Read the model definition and answer for the solid it produces. Units are mm, in the model's axes. A direction names the side the tool comes from. Coordinates: 2 decimals unless noted, no trailing zeros. Loops run counter-clockwise (first coordinate to the right, second up) from the corner with the lowest first, then second, coordinate; pieces in that order, holes last.
from build123d import *

# Parameters (mm, degrees)
SKETCH1_W           = 31
SKETCH1_H           = 45.4
BOSS_EXTRUDE1_DEPTH = 12
SKETCH2_W           = 27
SKETCH2_H           = 10
CUT_EXTRUDE1_DEPTH  = 57.268641356
SKETCH3_R           = 1.6
CUT_EXTRUDE2_DEPTH  = 10
SKETCH4_W           = 15
SKETCH4_H           = 12
BOSS_EXTRUDE2_DEPTH = 15
SKETCH5_R           = 1.6
CUT_EXTRUDE3_DEPTH  = 20
FILLET1_R           = 5
BOSS_EXTRUDE3_DEPTH = 15
CHAMFER1_SIZE       = 5
CUT_EXTRUDE4_DEPTH  = 4


with BuildPart() as part:
    # Sketch1 → Boss-Extrude1 (new body)
    with BuildSketch(Plane(origin=(0, 0, 0), x_dir=(1, 0, 0), z_dir=(0, 1, 0))):
        with Locations((15.5, 22.7)):
            Rectangle(SKETCH1_W, SKETCH1_H)
    extrude(amount=BOSS_EXTRUDE1_DEPTH)

    # Sketch2 → Cut-Extrude1 (cut, through all)
    with BuildSketch(Plane.XY):
        with Locations((15.5, 5)):
            Rectangle(SKETCH2_W, SKETCH2_H)
    extrude(amount=-CUT_EXTRUDE1_DEPTH, mode=Mode.SUBTRACT)

    # Sketch3 → Cut-Extrude2 (cut)
    with BuildSketch(Plane(origin=(0, 12, 0), x_dir=(1, 0, 0), z_dir=(0, 1, 0))):
        with Locations(Location((5.5, 32.7, 0), (0, 0, 270))):
            Circle(SKETCH3_R)
        with Locations(Location((25.5, 32.7, 0), (0, 0, 270))):
            Circle(SKETCH3_R)
        with Locations(Location((25.5, 12.7, 0), (0, 0, 270))):
            Circle(SKETCH3_R)
        with Locations(Location((5.5, 12.7, 0), (0, 0, 270))):
            Circle(SKETCH3_R)
    extrude(amount=-CUT_EXTRUDE2_DEPTH, mode=Mode.SUBTRACT)

    # Sketch4 → Boss-Extrude2 (add)
    with BuildSketch(Plane.ZY):
        with Locations((-7.5, 6)):
            Rectangle(SKETCH4_W, SKETCH4_H)
    extrude(amount=BOSS_EXTRUDE2_DEPTH)

    # Sketch5 → Cut-Extrude3 (cut)
    with BuildSketch(Plane(origin=(0, 12, 0), x_dir=(1, 0, 0), z_dir=(0, 1, 0))):
        with Locations(Location((-10, 5, 0), (0, 0, 270))):
            Circle(SKETCH5_R)
    extrude(amount=-CUT_EXTRUDE3_DEPTH, mode=Mode.SUBTRACT)

    # Fillet1
    fillet1_edges = [part.edges().sort_by_distance(p)[0] for p in [
        (-15, 6, -15),
        (-15, 6, 0),
    ]]
    fillet(fillet1_edges, radius=FILLET1_R)

    # Sketch6 → Boss-Extrude3 (add)
    with BuildSketch(Plane(origin=(31, 0, 0), x_dir=(0, 0, -1), z_dir=(1, 0, 0))):
        Polygon((5, 0), (10, 0), (10, 4.7), (25, 4.7), (25, 0), (30, 0), (30, 12), (5, 12), align=None)
    extrude(amount=BOSS_EXTRUDE3_DEPTH)

    # Chamfer1
    chamfer1_edges = [part.edges().sort_by_distance(p)[0] for p in [
        (38.5, 0, -5),
        (38.5, 0, -30),
    ]]
    chamfer(chamfer1_edges, length=CHAMFER1_SIZE - 0.0001)  # a hair under: the kernel refuses the full size

    # Sketch7 → Cut-Extrude4 (cut)
    with BuildSketch(Plane(origin=(43, 0, 0), x_dir=(0, 0, -1), z_dir=(1, 0, 0))):
        Polygon((5, 7), (15, 12), (5, 12), align=None)
        Polygon((30, 7), (20, 12), (30, 12), align=None)
    extrude(amount=-CUT_EXTRUDE4_DEPTH, mode=Mode.SUBTRACT)


with BuildPart() as body_2:
    # Mirror2: mirrored copy
    add(part.part.mirror(Plane(origin=(31, 12, 0), x_dir=(0, 0, 1), z_dir=(-1, 0, 0))))


with BuildPart() as body_3:
    # Mirror3: mirrored copy
    add(body_2.part.mirror(Plane(origin=(62, 12, -45.4), x_dir=(1, 0, 0), z_dir=(0, 0, 1))))


solid = body_3.part
Item 1: Find the intervals of material crossed by line 1 along Z through (x, y) = (36.5, 11.5); line 2 along X through (y, z) = (9.5, -64); line 3 along X through (y, z) = (2.75, -68.5), in increasing order.
Numbers:
line 1: z = -90.8 to -79.7, -76.5 to -59.7, -56.5 to -45.4
line 2: x = 16 to 19, 23 to 33, 60 to 62
line 3: x = 31 to 33, 60 to 62
Item 2: A cutting plane is placed at A-A on x = 56.5. Determine the outline of the cut face in (y, z), then the cut area to 3 significant figures.
Numbers:
outline: (10, -90.8) - (12, -90.8) - (12, -79.7) - (10, -79.7) - close; (10, -76.5) - (12, -76.5) - (12, -59.7) - (10, -59.7) - close; (10, -56.5) - (12, -56.5) - (12, -45.4) - (10, -45.4) - close
area: 78.0 mm2
Item 3: Which of the six approach directions +Z, -Z, +X, -X, +Y, -Y give full straight-line access (tool end or side, diameter ignored) to faces 1 (the face through (24, 8, -60.8)), 2 (the face through (20.972, 9.465, -65.73)), 3 (the face through (23.6, 2.5, -63.3)), 4 (the face through (23.6, 2.5, -83.3))?
Numbers:
face 1: +Z, -X, +Y, -Y
face 2: +Z, +Y
face 3: +Z, -X, -Y
face 4: -Z, -X, -Y
Item 4: A cutting plane is placed at B-B on z = -74.5. Determine the outline of the cut face in (x, y), then the cut area to 4 significant figures.
Numbers:
outline: (16, 4.7) - (31, 4.7) - (31, 0) - (33, 0) - (33, 10) - (60, 10) - (60, 0) - (62, 0) - (62, 12) - (16, 12) - close
area: 211.5 mm2
Item 5: Determine the mould class of faces 5 (the face through (75.57, 6.08, -89.3)), 6 (the face through (60, 5, -68)), 7 (the face through (45.4, 10.4, -45.4)), 8 (the face through (56.019, 11.014, -79.626)) for opening direction X: released by +X, released by -X, zero draft, split by the parting line, or undercut.
Numbers:
face 5: released by +X
face 6: undercut
face 7: zero draft
face 8: undercut
Item 6: Given pin 1 (2.5 mm diameter, centred on x = 24, y = 3, fed in from -Z); pin 2 (1.9 mm diameter, centred on x = 36.5, z = -78.1, fed in from -Y); pin 3 (5 mm diameter, centred on x = 69, y = 7.5, fed in from +Z); pin 4 (5 mm diameter, centred on x = 23, y = 3, fed in from +Z), each flat-ended and moving along its own axis, determine where each tip first touches the part or whether it passes through.
Numbers:
pin 1: stops at z = -85.05
pin 2: passes through
pin 3: stops at z = -75.8
pin 4: stops at z = -60.8
Item 7: A cutting plane is placed at C-C on z = -59. Determine the outline of the cut face in (x, y).
Numbers:
outline: (31, 0) - (33, 0) - (33, 10) - (35.18, 10) - (35.18, 12) - (31, 12) - close; (37.82, 10) - (55.18, 10) - (55.18, 12) - (37.82, 12) - close; (57.82, 10) - (60, 10) - (60, 0) - (62, 0) - (62, 12) - (57.82, 12) - close
